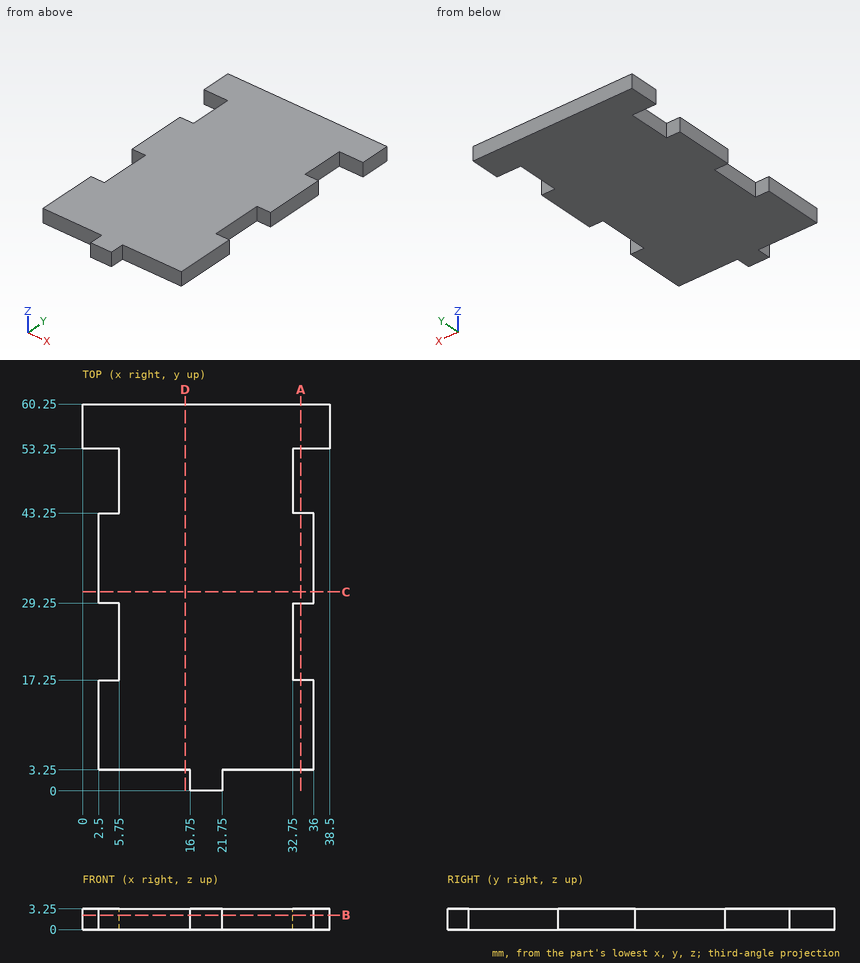
Geometry: see drawing. Coordinates: mm, zero at the bounding-box minimum. Round coordinates to 2 decimals unless told otherwise and drop trailing zeros. Write each loop counter-clockwise with the first axis right and the second up, starting at its lowest first coordinate (ties: lowest second). Pieces come first, ordered by that corner, then holes.
Item 1: Section query A-A (x = 34). Return loops of the section in (y, z), plus the area to 3 significant figures.
Item 2: Section query B-B (z = 2.25). Return loops of the section in (x, y), plus the area to 3 significant figures.
Item 3: Pin query (flat end, axial travel): P1, Ø1.6, axis at y = 36.5, z = 1, coming from the -X side; P2, Ø1, axis at y = 22, z = 2, coming from the +X side; P3, Ø1, axis at y = 1.5, z = 1, coming from the +X side. Return the tip coordinate at first contact, or that it passes through.
Item 4: Material intervals for L1, parallel to Y at x = 4.5, z = 1.6; L2, parallel to Y at x = 29, z = 0.45; L3, parallel to X at y = 34, z = 0.1, sorted ascending.
Item 5: Section query C-C (y = 31). Return loops of the section in (x, z), plus the area to 3 significant figures.
Item 6: Section query D-D (x = 16). Return loops of the section in (y, z), plus the area to 3 significant figures.
Completed:
1. outline: (3.25, 0) - (17.25, 0) - (17.25, 3.25) - (3.25, 3.25) - close; (29.25, 0) - (43.25, 0) - (43.25, 3.25) - (29.25, 3.25) - close; (53.25, 0) - (60.25, 0) - (60.25, 3.25) - (53.25, 3.25) - close
1. area: 114 mm2
2. outline: (0, 53.25) - (5.75, 53.25) - (5.75, 43.25) - (2.5, 43.25) - (2.5, 29.25) - (5.75, 29.25) - (5.75, 17.25) - (2.5, 17.25) - (2.5, 3.25) - (16.75, 3.25) - (16.75, 0) - (21.75, 0) - (21.75, 3.25) - (36, 3.25) - (36, 17.25) - (32.75, 17.25) - (32.75, 29.25) - (36, 29.25) - (36, 43.25) - (32.75, 43.25) - (32.75, 53.25) - (38.5, 53.25) - (38.5, 60.25) - (0, 60.25) - close
2. area: 1,820 mm2
3. P1: stops at x = 2.5
3. P2: stops at x = 32.75
3. P3: stops at x = 21.75
4. L1: y = 3.25 to 17.25, 29.25 to 43.25, 53.25 to 60.25
4. L2: y = 3.25 to 60.25
4. L3: x = 2.5 to 36
5. outline: (2.5, 0) - (36, 0) - (36, 3.25) - (2.5, 3.25) - close
5. area: 109 mm2
6. outline: (3.25, 0) - (60.25, 0) - (60.25, 3.25) - (3.25, 3.25) - close
6. area: 185 mm2
